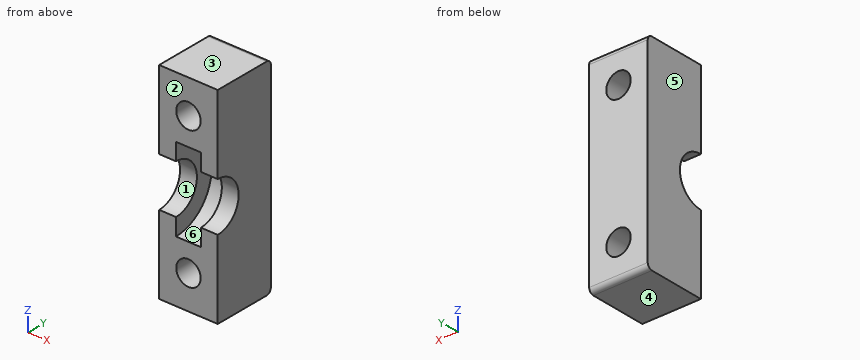
```python
from build123d import *

# Parameters (mm, degrees)
BOSS_EXTRUDE1_DEPTH = 12
SKETCH2_R           = 8.5
CUT_EXTRUDE1_DEPTH  = 2.55
CUT_EXTRUDE2_REACH  = 111.203
SKETCH3_R           = 2.5
FILLET1_R           = 1


with BuildPart() as part:
    # Sketch1 → Boss-Extrude1 (new body)
    with BuildSketch(Plane(origin=(100, 0, 0), x_dir=(0, 0, -1), z_dir=(1, 0, 0))):
        with BuildLine():
            Line((0, 23), (0, 35.7))
            Line((0, 35.7), (42, 35.7))
            Line((42, 35.7), (42, 23))
            Line((42, 23), (26, 23))
            ThreePointArc((26, 23), (21, 28), (16, 23))
            Line((16, 23), (0, 23))
        make_face()
    extrude(amount=-BOSS_EXTRUDE1_DEPTH)

    # Sketch2 → Cut-Extrude1 (cut, symmetric)
    with BuildSketch(Plane(origin=(94, 0, 0), x_dir=(0, 0, -1), z_dir=(1, 0, 0))):
        with Locations((21, 23)):
            Circle(SKETCH2_R)
    extrude(amount=CUT_EXTRUDE1_DEPTH, both=True, mode=Mode.SUBTRACT)

    # Sketch3 → Cut-Extrude2 (cut, up to next)
    with BuildSketch(Plane(origin=(0, 35.7, 0), x_dir=(1, 0, 0), z_dir=(0, 1, 0)), mode=Mode.PRIVATE) as cut_extrude2_sk1:
        with Locations(Location((94, 35.1, 0), (0, 0, 270))):
            Circle(SKETCH3_R)
    cut_extrude2_tool1 = extrude(cut_extrude2_sk1.sketch, amount=-CUT_EXTRUDE2_REACH, mode=Mode.PRIVATE) & part.part
    # Sketch3 → Cut-Extrude2 (cut, up to next)
    with BuildSketch(Plane(origin=(0, 35.7, 0), x_dir=(1, 0, 0), z_dir=(0, 1, 0)), mode=Mode.PRIVATE) as cut_extrude2_sk2:
        with Locations(Location((94, 6.9, 0), (0, 0, 270))):
            Circle(SKETCH3_R)
    cut_extrude2_tool2 = extrude(cut_extrude2_sk2.sketch, amount=-CUT_EXTRUDE2_REACH, mode=Mode.PRIVATE) & part.part
    add(cut_extrude2_tool1.solids().sort_by_distance((94, 35.7, -35.1))[0], mode=Mode.SUBTRACT)
    add(cut_extrude2_tool2.solids().sort_by_distance((94, 35.7, -6.9))[0], mode=Mode.SUBTRACT)

    # Fillet1
    fillet1_edges = [part.edges().sort_by_distance(p)[0] for p in [
        (94, 35.7, 0),
        (94, 35.7, -42),
    ]]
    fillet(fillet1_edges, radius=FILLET1_R)


solid = part.part
```
The listing builds one solid part. Answer for the finished solid, in the listing's coordinates (mm). Face numbers are marked on the shaded views. A direction names the side the tool comes from. Round coordinates to 2 decimals unless told otherwise and drop trailing zeros. Write each loop counter-clockwise with the first axis right and the second up, starting at its lowest first coordinate (ties: lowest second). Pieces come first, ordered by that corner, then holes. Notation, with made-up numbers: (61.5, 85) -> (87.5, 85) arc R32 cw to (87.5, 120) -> close; hole circle Ø6 at (76.25, 31). An arc over 180 degrees is marked (long way). Use CSV: the item, a comma, the result in double quotes. Start each with the question number.
(1) Section C-C on z = -6.9 is taken. Give the vertices of the cut face in (x, y).
(2) The mould has two halves that part along Z. Classify the marked faces 1, 2, 3 and 4: released by +Z, released by -Z, zero draft, split by the parting line, or undercut.
(3) Section D-D on y = 33.5 is taken. Give the vertices of the cut face in (x, z), then the cut area to 3 significant figures.
(4) Section B-B on y = 25.25 is taken. Give the vertices of the cut face in (x, z), then the cut area to 3 significant figures.
(5) This flat-tipped pin is pushed along its axis until it touches: pin 1 (4 mm diameter, centred on x = 94, z = -6.9, fed in from +Y). Where does it stop, or does it pass through?
(6) Section A-A on x = 94 is taken. Give the vertices of the cut face in (y, z).
(7) Which of the six approach directions +Z, -Z, +X, -X, +Y, -Y give full straight-line access (tool end or side, diameter ignored) to the marked faces 5 and 6?
(8) Consider L1, parallel to X at y = 28.5, z = -6.9; L2, parallel to Z at x = 94.5, y = 26; L3, parallel to X at y = 30.25, z = -8 (3 decimals). Determine where each line is inside the solid, lowest interval first. Write a range as from..to.
A:
1,outline,"(88, 23) -> (91.5, 23) -> (91.5, 35.7) -> (88, 35.7) -> close; (96.5, 23) -> (100, 23) -> (100, 35.7) -> (96.5, 35.7) -> close"
2,face 1,"undercut"
2,face 2,"zero draft"
2,face 3,"released by +Z"
2,face 4,"released by -Z"
3,outline,"(88, -42) -> (100, -42) -> (100, 0) -> (88, 0) -> close; hole circle Ø5 at (94, -35.1); hole circle Ø5 at (94, -6.9)"
3,area,"465 mm²"
4,outline,"(88, -42) -> (100, -42) -> (100, -25.47) -> (96.55, -25.47) -> (96.55, -29.2) -> (91.45, -29.2) -> (91.45, -25.47) -> (88, -25.47) -> close; (88, -16.53) -> (91.45, -16.53) -> (91.45, -12.8) -> (96.55, -12.8) -> (96.55, -16.53) -> (100, -16.53) -> (100, 0) -> (88, 0) -> close; hole circle Ø5 at (94, -35.1); hole circle Ø5 at (94, -6.9)"
4,area,"320 mm²"
5,pin 1,"passes through"
6,outline,"(23, -42) -> (34.7, -42) arc R1 ccw to (35.7, -41) -> (35.7, -37.6) -> (23, -37.6) -> close; (23, -32.6) -> (35.7, -32.6) -> (35.7, -9.4) -> (23, -9.4) -> (23, -12.5) arc R8.5 cw to (23, -29.5) -> close; (23, -4.4) -> (35.7, -4.4) -> (35.7, -1) arc R1 ccw to (34.7, 0) -> (23, 0) -> close"
7,face 5,"+Z, -Z, -X, +Y, -Y"
7,face 6,"-Y"
8,L1,"x = 88..91.5, 96.5..100"
8,L2,"z = -42..-37.55, -32.65..-28.95, -13.05..-9.35, -4.45..0"
8,L3,"x = 88..91.755, 96.245..100"
